The listing builds one solid part. Answer for the finished solid, in the listing's coordinates (mm). A direction names the side the tool comes from. Round coordinates to 2 decimals unless told otherwise and drop trailing zeros. Loops run counter-clockwise (first coordinate to the right, second up) from the corner with the lowest first, then second, coordinate; pieces in that order, holes last. Notation, with made-up numbers: (-34.5, -39) -> (21.5, -39) arc R26 cw to (21.5, -16) -> close; hole circle Ø11 at (-8, -22). An arc over 180 degrees is marked (long way). Answer in a Markdown table with one row per item. Add a question column.
```python
from build123d import *

# Parameters (mm, degrees)
SKETCH1_W           = 47
SKETCH1_H           = 26.5
SKETCH1_W_2         = 41
SKETCH1_H_2         = 20.5
BOSS_EXTRUDE1_DEPTH = 31
CUT_EXTRUDE2_DEPTH  = 31
SKETCH4_W           = 10
SKETCH4_H           = 10
BOSS_EXTRUDE3_DEPTH = 100
SKETCH7_R           = 2.9
CUT_EXTRUDE5_DEPTH  = 100
SKETCH8_R           = 7.284546015
SKETCH8_R_2         = 2.9
BOSS_EXTRUDE4_DEPTH = 10
SKETCH10_W          = 26.5
SKETCH10_H          = 7.496145738
CUT_EXTRUDE6_DEPTH  = 105


with BuildPart() as part:
    # Sketch1 → Boss-Extrude1 (new body)
    with BuildSketch(Plane(origin=(0, 0, 0), x_dir=(1, 0, 0), z_dir=(0, 1, 0))):
        Rectangle(SKETCH1_W, SKETCH1_H)
        Rectangle(SKETCH1_W_2, SKETCH1_H_2, mode=Mode.SUBTRACT)
    extrude(amount=BOSS_EXTRUDE1_DEPTH)

    # Sketch3 → Cut-Extrude2 (cut)
    with BuildSketch(Plane(origin=(0, 31, 0), x_dir=(1, 0, 0), z_dir=(0, 1, 0))):
        Polygon((-19.366144394, -10.25), (-20.5, -13.25), (0, -13.25), (0, -10.25), align=None)
        Polygon((0, -10.25), (0, -13.25), (20.5, -13.25), (19.366144394, -10.25), align=None)
    extrude(amount=-CUT_EXTRUDE2_DEPTH, mode=Mode.SUBTRACT)

    # Sketch4 → Boss-Extrude3 (add)
    with BuildSketch(Plane(origin=(0, 0, -13.25), x_dir=(-1, 0, 0), z_dir=(0, 0, -1))):
        with Locations((0, 26)):
            Rectangle(SKETCH4_W, SKETCH4_H)
    extrude(amount=BOSS_EXTRUDE3_DEPTH)

    # Sketch7 → Cut-Extrude5 (cut)
    with BuildSketch(Plane.XZ.offset(-21)):
        with Locations(Location((0, -88.166602936, 0), (0, 0, 270))):
            Circle(SKETCH7_R)
    extrude(amount=-CUT_EXTRUDE5_DEPTH, mode=Mode.SUBTRACT)

    # Sketch8 → Boss-Extrude4 (add)
    with BuildSketch(Plane(origin=(0, 21, 0), x_dir=(-1, 0, 0), z_dir=(0, -1, 0))):
        with Locations((0, 88.166602936)):
            Circle(SKETCH8_R)
        with Locations(Location((0, 88.166602936, 0), (0, 0, 90))):
            Circle(SKETCH8_R_2, mode=Mode.SUBTRACT)
    extrude(amount=-BOSS_EXTRUDE4_DEPTH)

    # Sketch10 → Cut-Extrude6 (cut)
    with BuildSketch(Plane.ZY.offset(23.5)):
        with Locations((0, 3.748072869)):
            Rectangle(SKETCH10_W, SKETCH10_H)
    extrude(amount=-CUT_EXTRUDE6_DEPTH, mode=Mode.SUBTRACT)


solid = part.part
```
Item 1: Consider L1, parallel to X at y = 26, z = 1.5; L2, parallel to Z at x = -8, y = 15.25; L3, parallel to X at y = 25.25, z = -61. Determine where each line is inside the solid, lowest interval first. Write a range as from..to.
Item 2: For faces 1 (the flat face through (-5, 26, -48)), 2 (the flat face through (0, 21, -64)), 3 (the flat face through (5, 26, -103)), 4 (the flat face through (-20.5, 19, 0)), 5 (the flat face through (5, 26, -48)), determine the directions among +Z, -Z, +X, -X, +Y, -Y from which every point of the face is accessible in a straight line to the end or side of a thin tool.
Item 3: Section C-C, the plane x = -10 is taken. Write down the section's boundary in (y, z), and give its area (3 significant figures).
Item 4: The mould has two halves that part along Z. Classify faces 6 (the cylindrical face through (-7.284, 25.93, -88.084)), 7 (the flat face through (-19.925, 19.413, 11.729)), 8 (the flat face through (-5, 26, -103)): +Z half, -Z half, draft (parallel to the pull), parting line (faces both ways), or undercut.
Item 5: Section A-A, the plane x = 0 is taken. Write down the section's boundary in (y, z).
Item 6: Section B-B, the plane y = 13 is taken. Write down the section's boundary in (x, z).
Item 7: Flat-ended cylindrical pins translate along their axes: P1, Ø11, axis at y = 27, z = -54, coming from the -X side; P2, Ø6, axis at x = 10.5, y = 27.5, coming from the -Z side; P3, Ø1, axis at y = 23.5, z = -86.5, coming from the -X side; P4, Ø4, axis at x = 5, z = -8.5, coming from the +Y side. Find the tip coordinate at first contact, or state that the pin passes through.
Here are the results:
| question | item | result |
|---|---|---|
| 1 | L1 | x = -23.5..-20.5, 20.5..23.5 |
| 1 | L2 | z = -13.25..-10.25 |
| 1 | L3 | x = -5..5 |
| 2 | face 1 | -X, +Y, -Y |
| 2 | face 2 | -Z, +X, -X, -Y |
| 2 | face 3 | -Z, +X, +Y, -Y |
| 2 | face 4 | +Y, -Y |
| 2 | face 5 | +X, +Y, -Y |
| 3 | outline | (7.5, -13.25) -> (31, -13.25) -> (31, -10.25) -> (7.5, -10.25) -> close |
| 3 | area | 70.5 mm² |
| 4 | face 6 | undercut |
| 4 | face 7 | +Z half |
| 4 | face 8 | draft |
| 5 | outline | (7.5, -13.25) -> (21, -13.25) -> (21, -85.27) -> (31, -85.27) -> (31, -10.25) -> (7.5, -10.25) -> close; (21, -113.25) -> (31, -113.25) -> (31, -91.07) -> (21, -91.07) -> close |
| 6 | outline | (-23.5, -13.25) -> (23.5, -13.25) -> (23.5, 13.25) -> (20.5, 13.25) -> (19.37, 10.25) -> (20.5, 10.25) -> (20.5, -10.25) -> (-20.5, -10.25) -> (-20.5, 10.25) -> (-19.37, 10.25) -> (-20.5, 13.25) -> (-23.5, 13.25) -> close |
| 7 | P1 | stops at x = -5 |
| 7 | P2 | stops at z = -13.25 |
| 7 | P3 | stops at x = -7.19 |
| 7 | P4 | stops at y = 31 |
